```python
from build123d import *

# Parameters (mm, degrees)
ESQUISSE1_W             = 340
ESQUISSE1_H             = 148
BOSS_EXTRU_1_DEPTH      = 6
ESQUISSE2_W             = 6
ESQUISSE2_H             = 10
ESQUISSE2_H_2           = 35
ESQUISSE2_H_3           = 18
ESQUISSE2_W_2           = 68
ESQUISSE2_H_4           = 6
ESQUISSE2_H_5           = 34
ESQUISSE2_W_3           = 40
ENL_V_MAT_EXTRU_1_DEPTH = 6
ESQUISSE3_W             = 6
ESQUISSE3_H             = 20
ESQUISSE3_W_2           = 30
ESQUISSE3_H_2           = 15
ESQUISSE3_W_3           = 20
ESQUISSE3_H_3           = 6
ENL_V_MAT_EXTRU_2_DEPTH = 10
ESQUISSE4_R             = 1.5
ESQUISSE4_W             = 10
ESQUISSE4_H             = 6
ENL_V_MAT_EXTRU_3_DEPTH = 10
ESQUISSE7_W             = 328
ESQUISSE7_H             = 6
BOSS_EXTRU_2_DEPTH      = 17
ESQUISSE8_R             = 1.5
ESQUISSE8_W             = 10
ESQUISSE8_H             = 10
ENL_V_MAT_EXTRU_5_DEPTH = 371.863856422
ESQUISSE9_R             = 2.995
ESQUISSE9_R_2           = 3
ENL_V_MAT_EXTRU_8_DEPTH = 3
ESQUISSE10_W            = 14
ESQUISSE10_H            = 6
ESQUISSE10_W_2          = 10
ESQUISSE10_W_3          = 75
ESQUISSE10_H_2          = 4
ESQUISSE10_W_4          = 6
ESQUISSE10_H_3          = 21
ENL_V_MAT_EXTRU_9_DEPTH = 371.863856422


with BuildPart() as part:
    # Esquisse1 → Boss.-Extru.1 (new body)
    with BuildSketch(Plane.XY):
        with Locations((-170, 74)):
            Rectangle(ESQUISSE1_W, ESQUISSE1_H)
    extrude(amount=BOSS_EXTRU_1_DEPTH)

    # Esquisse2 → Enlèv. mat.-Extru.1 (cut)
    with BuildSketch(Plane.XY.offset(6)):
        Polygon((-272, 142), (-334, 142), (-334, 103), (-340, 103), (-340, 148), (-272, 148), align=None)
        Polygon((0, 148), (0, 118), (-6, 118), (-6, 142), (-35, 142), (-35, 148), align=None)
        with Locations((-3, 5)):
            Rectangle(ESQUISSE2_W, ESQUISSE2_H)
        with Locations((-337, 65.5)):
            Rectangle(ESQUISSE2_W, ESQUISSE2_H_2)
        with Locations((-337, 9)):
            Rectangle(ESQUISSE2_W, ESQUISSE2_H_3)
        with Locations((-170, 145)):
            Rectangle(ESQUISSE2_W_2, ESQUISSE2_H_4)
        with Locations((-3, 71)):
            Rectangle(ESQUISSE2_W, ESQUISSE2_H_5)
        with Locations((-84, 145)):
            Rectangle(ESQUISSE2_W_3, ESQUISSE2_H_4)
    extrude(amount=-ENL_V_MAT_EXTRU_1_DEPTH, mode=Mode.SUBTRACT)

    # Esquisse3 → Enlèv. mat.-Extru.2 (cut)
    with BuildSketch(Plane.XY.offset(6)):
        with Locations((-241, 42)):
            Rectangle(ESQUISSE3_W, ESQUISSE3_H)
        with Locations((-241, 102)):
            Rectangle(ESQUISSE3_W, ESQUISSE3_H)
        with Locations((-288.5, 70.5)):
            Rectangle(ESQUISSE3_W, ESQUISSE3_H)
        with Locations((-319, 134.5)):
            Rectangle(ESQUISSE3_W_2, ESQUISSE3_H_2)
        with Locations((-310, 31.5)):
            Rectangle(ESQUISSE3_W_3, ESQUISSE3_H_3)
    extrude(amount=-ENL_V_MAT_EXTRU_2_DEPTH, mode=Mode.SUBTRACT)

    # Esquisse4 → Enlèv. mat.-Extru.3 (cut)
    with BuildSketch(Plane.XY.offset(6)):
        with Locations((-151.5, 119)):
            Circle(ESQUISSE4_R)
        with Locations((-151.5, 7)):
            Circle(ESQUISSE4_R)
        with Locations((-169, 119)):
            Rectangle(ESQUISSE4_W, ESQUISSE4_H)
        with Locations((-134, 119)):
            Rectangle(ESQUISSE4_W, ESQUISSE4_H)
        with Locations((-134, 7)):
            Rectangle(ESQUISSE4_W, ESQUISSE4_H)
        with Locations((-169, 7)):
            Rectangle(ESQUISSE4_W, ESQUISSE4_H)
    extrude(amount=-ENL_V_MAT_EXTRU_3_DEPTH, mode=Mode.SUBTRACT)

    # Esquisse7 → Boss.-Extru.2 (add)
    with BuildSketch(Plane.XZ):
        with Locations((-170, 3)):
            Rectangle(ESQUISSE7_W, ESQUISSE7_H)
    extrude(amount=BOSS_EXTRU_2_DEPTH)

    # Esquisse8 → Enlèv. mat.-Extru.5 (cut, through all)
    with BuildSketch(Plane.XY.offset(6)):
        with Locations((-42, 145)):
            Circle(ESQUISSE8_R)
        with Locations((-129, 145)):
            Circle(ESQUISSE8_R)
        with Locations((-109, 145)):
            Circle(ESQUISSE8_R)
        with Locations((-3, 111)):
            Circle(ESQUISSE8_R)
        with Locations((-3, 95)):
            Circle(ESQUISSE8_R)
        with Locations((-3, 47)):
            Circle(ESQUISSE8_R)
        with Locations((-3, 17)):
            Circle(ESQUISSE8_R)
        with Locations((-122, 119)):
            Circle(ESQUISSE8_R)
        with Locations((-181, 119)):
            Circle(ESQUISSE8_R)
        with Locations((-122, 7)):
            Circle(ESQUISSE8_R)
        with Locations((-181, 7)):
            Circle(ESQUISSE8_R)
        with Locations((-211, 145)):
            Circle(ESQUISSE8_R)
        with Locations((-241, 145)):
            Circle(ESQUISSE8_R)
        with Locations((-241, 122)):
            Circle(ESQUISSE8_R)
        with Locations((-241, 82)):
            Circle(ESQUISSE8_R)
        with Locations((-241, 62)):
            Circle(ESQUISSE8_R)
        with Locations((-241, 22)):
            Circle(ESQUISSE8_R)
        with Locations((-241, -7)):
            Circle(ESQUISSE8_R)
        with Locations((-288.5, 87.5)):
            Circle(ESQUISSE8_R)
        with Locations((-288.5, 53.5)):
            Circle(ESQUISSE8_R)
        with Locations((-319.5, 123)):
            Circle(ESQUISSE8_R)
        with Locations((-293, 31.5)):
            Circle(ESQUISSE8_R)
        with Locations((-327, 31.5)):
            Circle(ESQUISSE8_R)
        with Locations((-337, 33)):
            Circle(ESQUISSE8_R)
        with Locations((-337, 93)):
            Circle(ESQUISSE8_R)
        with Locations((-329, -12)):
            Rectangle(ESQUISSE8_W, ESQUISSE8_H)
    extrude(amount=-ENL_V_MAT_EXTRU_5_DEPTH, mode=Mode.SUBTRACT)

    # Esquisse9 → Enlèv. mat.-Extru.8 (cut)
    with BuildSketch(Plane.XY.offset(6)):
        with Locations((-337, 33)):
            Circle(ESQUISSE9_R)
        with Locations((-327, 31.5)):
            Circle(ESQUISSE9_R_2)
        with Locations((-293, 31.5)):
            Circle(ESQUISSE9_R_2)
        with Locations((-288.5, 53.5)):
            Circle(ESQUISSE9_R_2)
        with Locations((-288.5, 87.5)):
            Circle(ESQUISSE9_R_2)
        with Locations((-241, 145)):
            Circle(ESQUISSE9_R)
        with Locations((-241, 122)):
            Circle(ESQUISSE9_R)
        with Locations((-241, 82)):
            Circle(ESQUISSE9_R)
        with Locations((-241, 62)):
            Circle(ESQUISSE9_R_2)
        with Locations((-241, 22)):
            Circle(ESQUISSE9_R_2)
        with Locations((-241, -7)):
            Circle(ESQUISSE9_R_2)
        with Locations((-211, 145)):
            Circle(ESQUISSE9_R)
        with Locations((-337, 93)):
            Circle(ESQUISSE9_R)
        with Locations((-181, 119)):
            Circle(ESQUISSE9_R)
        with Locations((-151.5, 119)):
            Circle(ESQUISSE9_R)
        with Locations((-129, 145)):
            Circle(ESQUISSE9_R)
        with Locations((-122, 119)):
            Circle(ESQUISSE9_R)
        with Locations((-109, 145)):
            Circle(ESQUISSE9_R)
        with Locations((-122, 7)):
            Circle(ESQUISSE9_R)
        with Locations((-151.5, 7)):
            Circle(ESQUISSE9_R)
        with Locations((-181, 7)):
            Circle(ESQUISSE9_R)
        with Locations((-42, 145)):
            Circle(ESQUISSE9_R)
        with Locations((-3, 111)):
            Circle(ESQUISSE9_R)
        with Locations((-3, 95)):
            Circle(ESQUISSE9_R)
        with Locations((-3, 47)):
            Circle(ESQUISSE9_R)
        with Locations((-3, 17)):
            Circle(ESQUISSE9_R)
    extrude(amount=-ENL_V_MAT_EXTRU_8_DEPTH, mode=Mode.SUBTRACT)

    # Esquisse10 → Enlèv. mat.-Extru.9 (cut, through all)
    with BuildSketch(Plane.XY.offset(6)):
        with Locations((-13, 57)):
            Rectangle(ESQUISSE10_W, ESQUISSE10_H)
        with Locations((-75, 57)):
            Rectangle(ESQUISSE10_W_2, ESQUISSE10_H)
        with Locations((-13, 7)):
            Rectangle(ESQUISSE10_W, ESQUISSE10_H)
        with Locations((-75, 7)):
            Rectangle(ESQUISSE10_W_2, ESQUISSE10_H)
        with Locations((-47.5, 43.5)):
            Rectangle(ESQUISSE10_W_3, ESQUISSE10_H_2)
        with Locations((-47.5, 32)):
            Rectangle(ESQUISSE10_W_3, ESQUISSE10_H_2)
        with Locations((-47.5, 20.5)):
            Rectangle(ESQUISSE10_W_3, ESQUISSE10_H_2)
        with Locations((-99.5, 32)):
            Rectangle(ESQUISSE10_W_4, ESQUISSE10_H_3)
    extrude(amount=-ENL_V_MAT_EXTRU_9_DEPTH, mode=Mode.SUBTRACT)


solid = part.part
```
The listing builds one solid part. Answer for the finished solid, in the listing's coordinates (mm). A direction names the side the tool comes from. Coordinates: 2 decimals unless noted, no trailing zeros. Write each loop counter-clockwise with the first axis right and the second up, starting at its lowest first coordinate (ties: lowest second). Pieces come first, ordered by that corner, then holes. Notation, with made-up numbers: (25.25, 44.25) - (49.25, 44.25) arc R17 cw to (49.25, 74.25) - close; hole circle Ø6 at (-3, -4.75). An arc over 180 degrees is marked (long way). Return JSON: item names as keys, results as strings. Group by question number.
1. A cutting plane is placed at C-C, the plane z = 0.95. Give the number of separate pieces and of enclosed holes in the cut face, plus the area to 3 significant figures.
2. Determine the mould class of faces 1 (the flat face through (-50, 148, 3)), 2 (the flat face through (-100, 21.5, 3)), 3 (the flat face through (-80, 57, 3)), 4 (the flat face through (0, 103, 3)) for opening direction X: released by +X, released by -X, zero draft, split by the parting line, or undercut.
3. Which of the six approach directions +Z, -Z, +X, -X, +Y, -Y give full straight-line access (tool end or side, diameter ignored) to faces 5 (the flat face through (-104, 145, 3)), 6 (the flat face through (-310, 28.5, 3)), 7 (the flat face through (-287, 52, 3))?
4. A cutting plane is placed at B-B, the plane x = -193. Determine the outline of the cut face in (y, z), plus the area to 3 significant figures.
5. A cutting plane is placed at A-A, the plane y = 74. Determine the outline of the cut face in (x, z), plus the area to 3 significant figures.
6. Given pin 1 (5 mm diameter, centred on x = -151.5, y = 7, fed in from +Z); pin 2 (1 mm diameter, centred on x = -305, z = 4.5, fed in from +Y); pin 3 (1.8 mm diameter, centred on x = -154, z = 2, fed in from +Y), each flat-ended and moving along its own axis, determine where each tip first touches the part or whether it passes through.
7. Straight lines are drawn through the part: L1, parallel to Y at x = -137, z = 1.15; L2, parallel to Y at x = -71, z = 0.65; L3, parallel to Y at x = -293, z = 3.7. For each, find the intervals that lie inside material, in ascending order.
Ans:
{
 "1": {"separate pieces": "1", "enclosed holes": "41", "area": "50,900 mm²"},
 "2": {"face 1": "zero draft", "face 2": "undercut", "face 3": "undercut", "face 4": "released by +X"},
 "3": {"face 5": "+Z, -Z, +Y", "face 6": "+Z, -Z", "face 7": "+Z"},
 "4": {"outline": "(-17, 0) - (142, 0) - (142, 6) - (-17, 6) - close", "area": "954 mm²"},
 "5": {"outline": "(-334, 0) - (-291.5, 0) - (-291.5, 6) - (-334, 6) - close; (-285.5, 0) - (-6, 0) - (-6, 6) - (-285.5, 6) - close", "area": "1,930 mm²"},
 "6": {"pin 1": "z = 3", "pin 2": "y = 127", "pin 3": "y = 142"},
 "7": {"L1": "-17 to 4, 10 to 116, 122 to 142", "L2": "-17 to 4, 10 to 18.5, 22.5 to 30, 34 to 41.5, 45.5 to 54, 60 to 142", "L3": "-17 to 28.5, 34.5 to 142"}
}
